Could you check a few things on this model? Use its own coordinates, in mm. A direction names the side the tool comes from. Round coordinates to 2 decimals unless told otherwise and drop trailing zeros. Write each loop counter-clockwise with the first axis right and the second up, starting at its lowest first coordinate (ties: lowest second). Pieces come first, ordered by that corner, then holes. Notation, with made-up numbers: (56.5, 63) -> (84.5, 63) arc R28 ccw to (84.5, 83) -> close; hole circle Ø3 at (-6, 65.25). An arc over 180 degrees is marked (long way). One line per question, with ' | ' between items. Start each with the question number.
1. For pin 1 Ø7 at (x, y) = (56.5, 1.5) entering from -Z; pin 2 Ø0.9 at (y, z) = (-16, -91) entering from -X; pin 3 Ø1.6 at (x, z) = (-128.5, -101) entering from -Y; pin 4 Ø0.9 at (x, y) = (-136, -16) entering from -Z, each with a flat end and sliding along its axis, tell me the tip position at first contact or that it passes through.
2. Imagine slicing it at C-C, the plane x = 111. List the corners of the cut face in (y, z) for me, and give its area (3 significant figures).
3. Thinking about a two-plate mould opening in X: for faces 1 (the cylindrical face through (60.747, 2.143, -86.308)), 2 (the flat face through (-142.5, 0, 1)), 3 (the flat face through (142.5, 0, 1)), 4 (the flat face through (93, 2, -108)), which applies, released by +X, released by -X, zero draft, split by the parting line, or undercut?
4. If I drill on line 1 along Y through (x, z) = (96, -78); line 2 along Z through (x, y) = (-12, 4); line 3 along Y through (x, z) = (128, 37.5), over which ranges is the centre line in solid material (lowest first)? Write a range as [from, to].
5. Imagine slicing it at A-A, the plane x = 35. List the corners of the cut face in (y, z) for me, and give its area (3 significant figures).
6. For faces 5 (the flat face through (31, 5, -104.7)), 6 (the flat face through (136, -17.1, -91)), 7 (the flat face through (-130.57, -0.054, -104.282)), which set-ups out of +Z, -Z, +X, -X, +Y, -Y let a thin tool reach every point of the face, with its end or its side?
7. Imagine slicing it at B-B, the plane z = 21.5. List the corners of the cut face in (x, y) for me.
from build123d import *

# Parameters (mm, degrees)
SKIZZE1_W                       = 200
SKIZZE1_H                       = 28
AUFSATZ_LINEAR_AUSTRAGEN1_DEPTH = 142.5
SKIZZE2_W                       = 15
SKIZZE2_H                       = 20.7
AUFSATZ_LINEAR_AUSTRAGEN2_DEPTH = 2
AUFSATZ_LINEAR_AUSTRAGEN3_DEPTH = 5
AUFSATZ_LINEAR_AUSTRAGEN4_DEPTH = 4.7
SKIZZE6_R                       = 4.5
AUFSATZ_LINEAR_AUSTRAGEN5_DEPTH = 3.3
SKIZZE7_R                       = 3.25
SCHNITT_LINEAR_AUSTRAGEN1_DEPTH = 44
SKIZZE8_W                       = 10
SKIZZE8_H                       = 10
AUFSATZ_LINEAR_AUSTRAGEN6_DEPTH = 3.1
SPIEGELN2_COPY_1_SKETCH_W       = 10
SPIEGELN2_COPY_1_SKETCH_H       = 10
SPIEGELN2_COPY_1_DEPTH          = 3.1


with BuildPart() as part:
    # Skizze1 → Aufsatz-Linear austragen1 (new, symmetric)
    with BuildSketch(Plane(origin=(0, 0, 0), x_dir=(0, 0, -1), z_dir=(1, 0, 0))):
        Rectangle(SKIZZE1_W, SKIZZE1_H)
    extrude(amount=AUFSATZ_LINEAR_AUSTRAGEN1_DEPTH, both=True)

    # Skizze2 → Aufsatz-Linear austragen2 (add)
    with BuildSketch(Plane(origin=(0, 0, -100), x_dir=(-1, 0, 0), z_dir=(0, 0, -1))):
        with Locations((130.5, 1.4)):
            Rectangle(SKIZZE2_W, SKIZZE2_H)
    extrude(amount=AUFSATZ_LINEAR_AUSTRAGEN2_DEPTH)

    # Skizze3 → Aufsatz-Linear austragen3 (add, symmetric)
    with BuildSketch(Plane.ZY.offset(130.5)):
        Polygon((-102, 9.25), (-106.5, 6.651923789), (-102, -6.95), align=None)
    extrude(amount=AUFSATZ_LINEAR_AUSTRAGEN3_DEPTH, both=True)

    # Skizze5 → Aufsatz-Linear austragen4 (add)
    with BuildSketch(Plane(origin=(0, 0, -100), x_dir=(-1, 0, 0), z_dir=(0, 0, -1))):
        Polygon((-100.830127019, -5.5), (-92.169872981, -5.5), (-87.839745962, 2), (-92.169872981, 9.5), (-100.830127019, 9.5), (-105.160254038, 2), align=None)
    aufsatz_linear_austragen4 = extrude(amount=AUFSATZ_LINEAR_AUSTRAGEN4_DEPTH)

    # Skizze6 → Aufsatz-Linear austragen5 (add)
    with BuildSketch(Plane(origin=(0, 0, -104.7), x_dir=(-1, 0, 0), z_dir=(0, 0, -1))):
        with Locations((-96.5, 2)):
            Circle(SKIZZE6_R)
    aufsatz_linear_austragen5 = extrude(amount=AUFSATZ_LINEAR_AUSTRAGEN5_DEPTH)

    # Skizze7 → Schnitt-Linear austragen1 (cut)
    with BuildSketch(Plane(origin=(0, 0, -108), x_dir=(-1, 0, 0), z_dir=(0, 0, -1))):
        with Locations((-96.5, 2)):
            Circle(SKIZZE7_R)
    schnitt_linear_austragen1 = extrude(amount=-SCHNITT_LINEAR_AUSTRAGEN1_DEPTH, mode=Mode.SUBTRACT)

    # Skizzen-Muster1: Aufsatz-Linear austragen4, Aufsatz-Linear austragen5, Schnitt-Linear austragen1 at 2 more places
    with Locations((-39, 0, 0), (-61.5, 0, 0)):
        add(aufsatz_linear_austragen4)
        add(aufsatz_linear_austragen5)
        add(schnitt_linear_austragen1, mode=Mode.SUBTRACT)

    # Skizze8 → Aufsatz-Linear austragen6 (add)
    with BuildSketch(Plane.XZ.offset(14)):
        with Locations((136.5, -91)):
            Rectangle(SKIZZE8_W, SKIZZE8_H)
    aufsatz_linear_austragen6 = extrude(amount=AUFSATZ_LINEAR_AUSTRAGEN6_DEPTH)

    # Spiegeln1: Aufsatz-Linear austragen6 across plane
    add(aufsatz_linear_austragen6.mirror(Plane(origin=(0, 0, 0), x_dir=(0, 0, 1), z_dir=(1, 0, 0))))

    # Spiegeln2: Aufsatz-Linear austragen6 across plane
    add(aufsatz_linear_austragen6.mirror(Plane.XY))

    # Spiegeln2 copy 1 sketch → Spiegeln2 copy 1 (add)
    with BuildSketch(Plane(origin=(0, -14, 0), x_dir=(-1, 0, 0), z_dir=(0, -1, 0))):
        with Locations((136.5, -91)):
            Rectangle(SPIEGELN2_COPY_1_SKETCH_W, SPIEGELN2_COPY_1_SKETCH_H)
    extrude(amount=SPIEGELN2_COPY_1_DEPTH)


solid = part.part
Geometry results:
1) pin 1: stops at z = -108 | pin 2: stops at x = -141.5 | pin 3: stops at y = -8.95 | pin 4: stops at z = -96
2) outline: (-14, -100) -> (14, -100) -> (14, 100) -> (-14, 100) -> close | area: 5,600 mm2
3) face 1: undercut | face 2: released by -X | face 3: released by +X | face 4: zero draft
4) line 1: y = [-14, -1.21], [5.21, 14] | line 2: z = [-100, 100] | line 3: y = [-14, 14]
5) outline: (-14, -100) -> (-5.5, -100) -> (-5.5, -104.7) -> (-2.5, -104.7) -> (-2.5, -108) -> (-1.25, -108) -> (-1.25, -64) -> (5.25, -64) -> (5.25, -108) -> (6.5, -108) -> (6.5, -104.7) -> (9.5, -104.7) -> (9.5, -100) -> (14, -100) -> (14, 100) -> (-14, 100) -> close | area: 5,410 mm2
6) face 5: -Z | face 6: +Z, -Z, +X, -X, -Y | face 7: -Z, -X, -Y
7) outline: (-142.5, -14) -> (142.5, -14) -> (142.5, 14) -> (-142.5, 14) -> close
